```python
from build123d import *

# Parameters (mm, degrees)
SKETCH1_R           = 7.8
BOSS_EXTRUDE1_DEPTH = 82.5
SKETCH2_W           = 33
SKETCH2_H           = 13
BOSS_EXTRUDE2_DEPTH = 1
SKETCH3_W           = 33
SKETCH3_H           = 3
BOSS_EXTRUDE3_DEPTH = 30


with BuildPart() as part:
    # Sketch1 → Boss-Extrude1 (new body)
    with BuildSketch(Plane.XY):
        Circle(SKETCH1_R)
    extrude(amount=BOSS_EXTRUDE1_DEPTH)

    # Sketch2 → Boss-Extrude2 (add)
    with BuildSketch(Plane(origin=(0, 0, 0), x_dir=(-1, 0, 0), z_dir=(0, 0, -1))):
        Rectangle(SKETCH2_W, SKETCH2_H)
    extrude(amount=-BOSS_EXTRUDE2_DEPTH)

    # Sketch3 → Boss-Extrude3 (add)
    with BuildSketch(Plane(origin=(0, 0, 0), x_dir=(-1, 0, 0), z_dir=(0, 0, -1))):
        Rectangle(SKETCH3_W, SKETCH3_H)
    extrude(amount=-BOSS_EXTRUDE3_DEPTH)


solid = part.part
```
Verification items for the finished model (mm, model axes). A direction names the side the tool comes from. Coordinates: 2 decimals unless noted, no trailing zeros. Write each loop counter-clockwise with the first axis right and the second up, starting at its lowest first coordinate (ties: lowest second). Pieces come first, ordered by that corner, then holes. Notation, with made-up numbers: M 63.25,-39.75 L 122.25,-39.75 A32 cw 122.25,-13.75 Z; hole C -25.5,76.25 d4. An arc over 180 degrees is marked long. Answer as a JSON object with one key per item and string values. Group by question number.
(1) Cross-section at B-B, the plane y = 0. Record the cut outline in (x, z).
(2) Release check for a two-part mould opening along X. For faces 5 (the face through (-12, 1.5, 15)), 6 (the face through (16.5, 0, 14)), 7 (the face through (7.44, 2.34, 40.67)) record: +X half, -X half, draft (parallel to the pull), parting line (faces both ways), or undercut.
(3) Gauge pin test, flat ends, axial feed: pin 1 (2.5 mm diameter, centred on x = -14, y = -0.5, fed in from +Z); pin 2 (8 mm diameter, centred on x = -11.5, y = -2.5, fed in from -Z); pin 3 (2.5 mm diameter, centred on x = 11, z = 8.5, fed in from +Y); pin 4 (0.5 mm diameter, centred on x = 10.5, z = 0.5, fed in from -Y). Record the tip position at first contact, or that the pin passes through.
(4) Tool access check on faces 1 (the face through (12, 1.5, 15)), 2 (the face through (12, -4, 1)), 3 (the face through (-12, 4, 1)), 4 (the face through (-12, -1.5, 15)). Record the directions out of +Z, -Z, +X, -X, +Y, -Y that give a thin tool (end or side, any length) a straight path to the whole face; none if there is none.
(5) Cross-section at C-C, the plane z = 58. Record the cut outline in (x, y), and give its area (3 significant figures).
(6) Cross-section at A-A, the plane z = 21. Record the cut outline in (x, y).
(7) Material ranges on line 1 (Z direction, x = 13, y = -3.75); line 2 (Y direction, x = -9.5, z = 27.5); line 3 (X direction, y = 2, z = 46), recorded low to high.
Reply:
{
 "1": {"outline": "M -16.5,0 L 16.5,0 L 16.5,30 L 7.8,30 L 7.8,82.5 L -7.8,82.5 L -7.8,30 L -16.5,30 Z"},
 "2": {"face 5": "draft", "face 6": "+X half", "face 7": "parting line"},
 "3": {"pin 1": "z = 30", "pin 2": "z = 0", "pin 3": "y = 1.5", "pin 4": "y = -6.5"},
 "4": {"face 1": "+Z, +X, +Y", "face 2": "+Z, +X, -Y", "face 3": "+Z, -X, +Y", "face 4": "+Z, -X, -Y"},
 "5": {"outline": "C 0,0 d15.6", "area": "191 mm²"},
 "6": {"outline": "M -16.5,-1.5 L -7.65,-1.5 A7.8 ccw 7.65,-1.5 L 16.5,-1.5 L 16.5,1.5 L 7.65,1.5 A7.8 ccw -7.65,1.5 L -16.5,1.5 Z"},
 "7": {"line 1": "0 to 1", "line 2": "-1.5 to 1.5", "line 3": "-7.54 to 7.54"}
}
